Design review of the part built by this model. Coordinates are the model's own, in mm. Face numbers are marked on the shaded views. A direction names the side the tool comes from. Give positions to 0.01 mm unless a question says otherwise; leave off trailing zeros. Order: outer loops, then holes, each group sorted by start corner. A loop starts at its lowest first (then second) coordinate and runs counter-clockwise, first axis right, second up. Notation, with made-up numbers: (27.5, 71) -> (57.5, 71) arc R24 ccw to (57.5, 95) -> close; hole circle Ø5 at (18.25, 58.5). An arc over 180 degrees is marked (long way). Return JSON: item names as keys, results as strings.
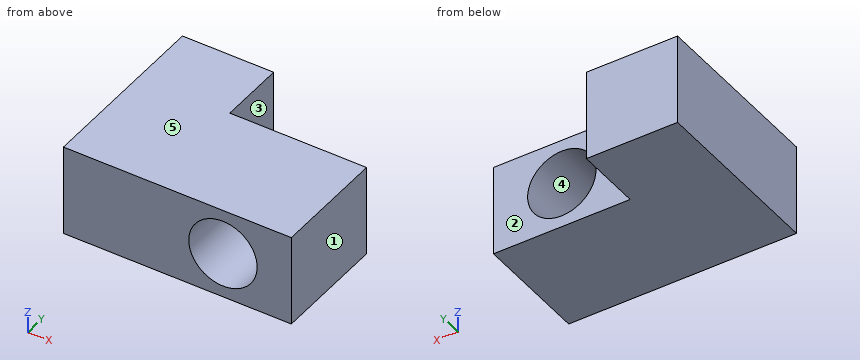
Autodesk Inventor part; units mm, degrees
ref_plane "YZ Plane" through (0, 0, 0) normal (1, 0, 0) x (0, 1, 0)
ref_plane "XZ Plane" through (0, 0, 0) normal (0, 1, 0) x (-1, 0, 0)
ref_plane "XY Plane" through (0, 0, 0) normal (0, 0, 1) x (1, 0, 0)
sketch "Sketch1" plane through (0, 0, 0) normal (0, 1, 0) x (-1, 0, 0)
  line L0 (0, 0) -> (-76.2, 0)
  line L1 (-76.2, 0) -> (-76.2, 50.8)
  line L2 (-76.2, 50.8) -> (0, 50.8)
  line L3 (0, 50.8) -> (0, 0)
  line L4 (0, 50.8) -> (50.8, 50.8)
  line L5 (50.8, 50.8) -> (50.8, 0)
  line L6 (50.8, 0) -> (0, 0)
  line L7 (0, 0) -> (0, 50.8)
  circle A0 centre (-38.1, 25.4) radius 19.05
  circle A1 centre (25.4, 37.0829) radius 6.964
  line L8 (50.8, 25.4) -> (-76.2, 25.4)
  point P0 (-57.15, 25.4)
  point P1 (-19.05, 25.4)
  point P2 (0, 25.4)
  dimension "d0" = 76.2
  dimension "d1" = 50.8
  dimension "d2" = 50.8
  dimension "d3" = 38.1
extrude "Extrusion3" add sketch "Sketch1" along normal blind 64.2112 contours L8 A0 L1 L2 L3
extrude "Extrusion4" add sketch "Sketch1" along normal blind 101.6 contours L3 L4 L5 L8 | A1
mirror "Mirror1" about plane through (76.2, 0, 25.4) normal (0, 0, -1)
properties part number "Cylinder Block"
Item 1: Mouldability with a two-part tool opening along X and no side actions: class the marked faces 3, 4 and 5 as released by +X, released by -X, zero draft, split by the parting line, or undercut.
Result set:
{"face 3": "released by +X", "face 4": "undercut", "face 5": "zero draft"}
Item 2: Add section A-A (z = 25.4). Give the boundary of the cut face in (x, y).
Result set:
{"outline": "(-50.8, 0) -> (19.05, 0) -> (19.05, 64.21) -> (0, 64.21) -> (0, 101.6) -> (-50.8, 101.6) -> close; (57.15, 0) -> (76.2, 0) -> (76.2, 64.21) -> (57.15, 64.21) -> close"}
Item 3: Machinability: for the marked faces 1 and 2, which of the approach directions +Z, -Z, +X, -X, +Y, -Y give a long, thin tool a straight path to every point of the face, cutting with its end or side? Answer none if there is none.
Result set:
{"face 1": "+Z, -Z, +X, +Y, -Y", "face 2": "+Z, -Z, +X, +Y"}
Item 4: For pin 1 (23 mm diameter, centred on x = 38.1, z = 25.4, fed in from +Y) (1 decimal); pin 2 (11 mm diameter, centred on y = 80, z = 25.5, fed in from +X); pin 3 (12 mm diameter, centred on x = 23, z = 29.5, fed in from +Y), all flat-tipped, find the tip position at first contact; note any pin that passes through.
Result set:
{"pin 1": "passes through", "pin 2": "stops at x = 0", "pin 3": "stops at y = 64.21"}
Item 5: Add section B-B (x = 38.1). Give the boundary of the cut face in (y, z).
Result set:
{"outline": "(0, 0) -> (64.21, 0) -> (64.21, 6.35) -> (0, 6.35) -> close; (0, 44.45) -> (64.21, 44.45) -> (64.21, 50.8) -> (0, 50.8) -> close"}
Item 6: Add section D-D (z = 9.5). Give the boundary of the cut face in (x, y).
Result set:
{"outline": "(-50.8, 0) -> (27.61, 0) -> (27.61, 64.21) -> (0, 64.21) -> (0, 101.6) -> (-50.8, 101.6) -> close; (48.59, 0) -> (76.2, 0) -> (76.2, 64.21) -> (48.59, 64.21) -> close"}
Item 7: Add section C-C (y = 46). Give the boundary of the cut face in (x, z).
Result set:
{"outline": "(-50.8, 0) -> (76.2, 0) -> (76.2, 50.8) -> (-50.8, 50.8) -> close; hole circle Ø38.1 at (38.1, 25.4)"}
Item 8: Wall thickness on L1, parallel to Z at x = 38, y = 30; L2, parallel to X at y = 41, z = 25; L3, parallel to X at y = 87, z = 46: over which ranges is each line inside the solid? List them lowest first. Write a range as [from, to].
Result set:
{"L1": "z = [0, 6.35], [44.45, 50.8]", "L2": "x = [-50.8, 19.05], [57.15, 76.2]", "L3": "x = [-50.8, 0]"}
